Design review of the part built by this model. Coordinates are the model's own, in mm. Face numbers are marked on the shaded views. A direction names the side the tool comes from. Coordinates: 2 decimals unless noted, no trailing zeros. Write each loop counter-clockwise with the first axis right and the second up, starting at its lowest first coordinate (ties: lowest second). Pieces come first, ordered by that corner, then holes. Notation, with made-up numbers: (65, -35.5) -> (87, -35.5) arc R19 ccw to (87, -3.5) -> close; hole circle Ø10 at (7.25, 25). An arc over 180 degrees is marked (long way). Answer in a Markdown table with one row per item. Add a question column.
Item 1: To check wall thickness, follow line 1 (X direction, y = 17.5, z = -21); line 2 (Z direction, x = 6, y = 6); line 3 (X direction, y = 18, z = 0). State the ranges of each line that lie inside material, in increasing order.
Item 2: Clearance check with flat-ended pins moving along their axes: P1, Ø1, axis at y = 8, z = -17.5, coming from the +X side; P2, Ø3, axis at x = 25, y = 7.5, coming from the -Z side; P3, Ø4, axis at x = -41, z = -6.5, coming from the +Y side; P4, Ø1.9, axis at y = 7.5, z = -15, coming from the +X side. State where each tip first meets the part, or that it passes through.
Item 3: Take a section at C-C, the plane x = 0. Give the number of separate pieces and of enclosed holes in the cut face, and give its area (3 significant figures).
Item 4: Draft analysis for pull direction X (two halves, no side actions). For the marked faces 6, 7 and 8, state which applies: released by +X, released by -X, zero draft, split by the parting line, or undercut.
Item 5: Take a section at B-B, the plane z = -20. Write out the cut boundary in (x, y).
Item 6: Take a section at D-D, the plane y = 27.5. Write out the cut boundary in (x, z), and give its area (3 significant figures).
Item 7: Take a section at A-A, the plane x = -50. Write out the cut boundary in (y, z).
Item 8: For the marked faces 1, 2, 3, 4 and 5, list the 3-axis set-ups (+Z, -Z, +X, -X, +Y, -Y) from which the entire face can be reached by the end or side of a thin tool; tool diameter is ignored.
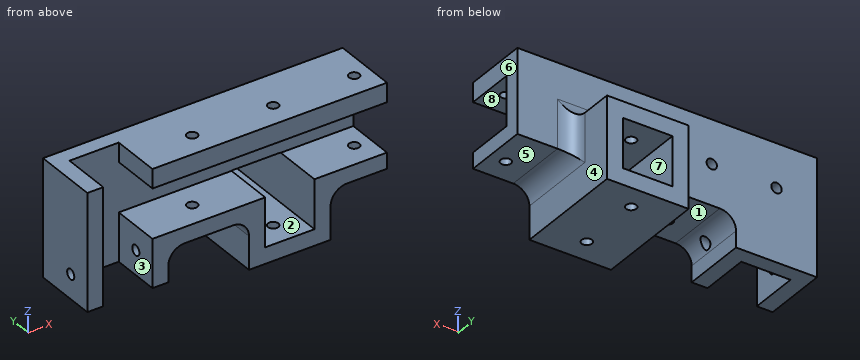
from build123d import *

# Parameters (mm, degrees)
SKETCH_1_W               = 15.2
SKETCH_1_H               = 15.2
EXTRUDE_1_DEPTH          = 20
SKETCH_2_W               = 25.2
SKETCH_2_H               = 25.2
SKETCH_2_W_2             = 15.2
SKETCH_2_H_2             = 15.2
EXTRUDE_2_DEPTH          = 15
SKETCH_3_W               = 15.2
SKETCH_3_H               = 15.2
CUT_EXTRUDE_1_DEPTH      = 80
SKETCH_4_R               = 1.6
CUT_EXTRUDE_2_DEPTH      = 83.635888087
FILLET_1_R               = 5
SKETCH_5_W               = 15.2
SKETCH_5_H               = 15.2
CUT_EXTRUDE_3_DEPTH      = 83.635888087
CUT_EXTRUDE_4_REACH      = 104.706
CUT_EXTRUDE_4_END_RADIUS = 5
SKETCH_6_R               = 1.6
CUT_EXTRUDE_5_REACH      = 73.229
SKETCH_7_R               = 1.6


with BuildPart() as part:
    # 草图1 → 凸台-拉伸1 (new body)
    with BuildSketch(Plane(origin=(0, 0, 0), x_dir=(1, 0, 0), z_dir=(0, 1, 0))):
        Polygon((-37.5, 12.5), (-12.6, 12.5), (-12.6, 27.7), (12.6, 27.7), (12.6, 12.5), (30, 12.5), (30, -13.5), (-62.5, -13.5), (-62.5, 22.5), (-37.5, 22.5), align=None)
        with Locations((0, 15.1)):
            Rectangle(SKETCH_1_W, SKETCH_1_H, mode=Mode.SUBTRACT)
    extrude(amount=EXTRUDE_1_DEPTH)

    # 草图2 → 凸台-拉伸2 (add)
    with BuildSketch(Plane(origin=(0, 20, 0), x_dir=(1, 0, 0), z_dir=(0, 1, 0))):
        with Locations((0, 15.1)):
            Rectangle(SKETCH_2_W, SKETCH_2_H)
        with Locations((0, 15.1)):
            Rectangle(SKETCH_2_W_2, SKETCH_2_H_2, mode=Mode.SUBTRACT)
    extrude(amount=EXTRUDE_2_DEPTH)

    # 草图3 → 切除-拉伸1 (cut)
    with BuildSketch(Plane(origin=(30, 0, 0), x_dir=(0, 0, -1), z_dir=(1, 0, 0))):
        with Locations((0, 7.6)):
            Rectangle(SKETCH_3_W, SKETCH_3_H)
    extrude(amount=-CUT_EXTRUDE_1_DEPTH, mode=Mode.SUBTRACT)

    # 草图4 → 切除-拉伸2 (cut, through all)
    with BuildSketch(Plane.XY.offset(13.5)):
        with Locations((0, 7.5)):
            Circle(SKETCH_4_R)
        with Locations((25, 7.5)):
            Circle(SKETCH_4_R)
        with Locations((-25, 7.5)):
            Circle(SKETCH_4_R)
        with Locations((0, 27.5)):
            Circle(SKETCH_4_R)
    extrude(amount=-CUT_EXTRUDE_2_DEPTH, mode=Mode.SUBTRACT)

    # 圆角1
    fillet_1_edges = [part.edges().sort_by_distance(p)[0] for p in [
        (-37.5, 10, -12.5),
        (-12.6, 10, -12.5),
        (12.6, 10, -12.5),
        (-12.6, 20, -7.5),
        (0, 20, -2.5),
        (12.6, 20, -7.5),
    ]]
    fillet(fillet_1_edges, radius=FILLET_1_R)

    # 草图5 → 切除-拉伸3 (cut, through all)
    with BuildSketch(Plane.XY.offset(13.5)):
        with Locations((-50, 7.6)):
            Rectangle(SKETCH_5_W, SKETCH_5_H)
    extrude(amount=-CUT_EXTRUDE_3_DEPTH, mode=Mode.SUBTRACT)

    # 切除-拉伸4: up to this cylinder (the profile starts outside it)
    cut_extrude_4_end = Plane(origin=(-32.5, 7.5, -17.5), z_dir=(0, 1, 0)) * Cylinder(CUT_EXTRUDE_4_END_RADIUS, 220.412, mode=Mode.PRIVATE)
    # 草图6 → 切除-拉伸4 (cut, up to the surface)
    with BuildSketch(Plane.ZY.offset(62.5), mode=Mode.PRIVATE) as cut_extrude_4_sk1:
        with Locations((-15, 7.5)):
            Circle(SKETCH_6_R)
    cut_extrude_4_tool1 = extrude(cut_extrude_4_sk1.sketch, amount=-CUT_EXTRUDE_4_REACH, mode=Mode.PRIVATE) - cut_extrude_4_end
    add(cut_extrude_4_tool1.solids().sort_by_distance((-62.5, 7.5, -15))[0], mode=Mode.SUBTRACT)

    # 草图7 → 切除-拉伸5 (cut, up to next)
    with BuildSketch(Plane(origin=(0, 20, 0), x_dir=(1, 0, 0), z_dir=(0, 1, 0)), mode=Mode.PRIVATE) as cut_extrude_5_sk1:
        with Locations(Location((-50, 0, 0), (0, 0, 270))):
            Circle(SKETCH_7_R)
    cut_extrude_5_tool1 = extrude(cut_extrude_5_sk1.sketch, amount=-CUT_EXTRUDE_5_REACH, mode=Mode.PRIVATE) & part.part
    # 草图7 → 切除-拉伸5 (cut, up to next)
    with BuildSketch(Plane(origin=(0, 20, 0), x_dir=(1, 0, 0), z_dir=(0, 1, 0)), mode=Mode.PRIVATE) as cut_extrude_5_sk2:
        with Locations(Location((-30, 0, 0), (0, 0, 270))):
            Circle(SKETCH_7_R)
    cut_extrude_5_tool2 = extrude(cut_extrude_5_sk2.sketch, amount=-CUT_EXTRUDE_5_REACH, mode=Mode.PRIVATE) & part.part
    add(cut_extrude_5_tool1.solids().sort_by_distance((-50, 20, 0))[0], mode=Mode.SUBTRACT)
    add(cut_extrude_5_tool2.solids().sort_by_distance((-30, 20, 0))[0], mode=Mode.SUBTRACT)


solid = part.part
Answers:
| question | item | result |
|---|---|---|
| 1 | line 1 | x = -62.5 to -37.5, -12.6 to -7.6, 7.6 to 12.6 |
| 1 | line 2 | z = -27.7 to -22.7, 7.6 to 13.5 |
| 1 | line 3 | x = -62.5 to -51.6, -48.4 to -31.6, -28.4 to 30 |
| 2 | P1 | stops at x = 12.63 |
| 2 | P2 | passes through |
| 2 | P3 | stops at y = 20 |
| 2 | P4 | stops at x = 13.98 |
| 3 | separate pieces | 6 |
| 3 | enclosed holes | 0 |
| 3 | area | 379 mm^2 |
| 4 | face 6 | released by +X |
| 4 | face 7 | undercut |
| 4 | face 8 | zero draft |
| 5 | outline | (-62.5, 0) -> (-57.6, 0) -> (-57.6, 15.2) -> (-42.4, 15.2) -> (-42.4, 0) -> (-37.5, 0) -> (-37.5, 20) -> (-62.5, 20) -> close; (-12.6, 0) -> (-7.6, 0) -> (-7.6, 35) -> (-12.6, 35) -> close; (7.6, 0) -> (12.6, 0) -> (12.6, 35) -> (7.6, 35) -> close |
| 6 | outline | (-12.6, -27.7) -> (-1.6, -27.7) -> (-1.6, -22.7) -> (-7.6, -22.7) -> (-7.6, -7.5) -> (-1.6, -7.5) -> (-1.6, -2.5) -> (-12.6, -2.5) -> close; (1.6, -27.7) -> (12.6, -27.7) -> (12.6, -2.5) -> (1.6, -2.5) -> (1.6, -7.5) -> (7.6, -7.5) -> (7.6, -22.7) -> (1.6, -22.7) -> close |
| 6 | area | 372 mm^2 |
| 7 | outline | (15.2, -22.5) -> (20, -22.5) -> (20, -1.6) -> (15.2, -1.6) -> close; (15.2, 1.6) -> (20, 1.6) -> (20, 13.5) -> (15.2, 13.5) -> close |
| 8 | face 1 | -Z, +Y, -Y |
| 8 | face 2 | +Y, -Y |
| 8 | face 3 | +Z, -Z, -Y |
| 8 | face 4 | -Z, +X, +Y |
| 8 | face 5 | -Z, +X, +Y, -Y |
